```python
from build123d import *

# Parameters (mm, degrees)
EXTRUDE_1_DEPTH   = 5
EXTRUDE_1_2_DEPTH = 5
EXTRUDE_1_3_DEPTH = 3
SKETCH_3_W        = 8
SKETCH_3_H        = 4.5
EXTRUDE_2_DEPTH   = 1
FILLET_1_R        = 2
FILLET_2_R        = 0.4
FILLET_3_R        = 0.4


with BuildPart() as part:
    # Эскиз1 → Extrude 1 (new body)
    with BuildSketch(Plane(origin=(0, 0, 0), x_dir=(1, 0, 0), z_dir=(0, 1, 0))):
        Polygon((3.047071049, 14.786951222), (5.547071049, 14.786951222), (5.547071049, 20.386951222), (-4.052928951, 20.386951222), (-4.052928951, 14.786951222), (-1.552928951, 14.786951222), (-1.552928951, 14.286951222), (3.047071049, 14.286951222), align=None)
        Polygon((2.247071049, 15.586951222), (4.747071049, 15.586951222), (4.747071049, 19.586951222), (-3.252928951, 19.586951222), (-3.252928951, 15.586951222), (-0.752928951, 15.586951222), (-0.752928951, 15.086951222), (2.247071049, 15.086951222), align=None, mode=Mode.SUBTRACT)
    extrude(amount=EXTRUDE_1_DEPTH)



with BuildPart() as body_2:
    # Эскиз1 → Extrude 1 2 (new body)
    with BuildSketch(Plane(origin=(0, 0, 0), x_dir=(1, 0, 0), z_dir=(0, 1, 0))):
        Polygon((-4.052928951, -12.613048778), (-4.052928951, -18.213048778), (5.547071049, -18.213048778), (5.547071049, -12.613048778), (3.047071049, -12.613048778), (3.047071049, -12.113048778), (-1.552928951, -12.113048778), (-1.552928951, -12.613048778), align=None)
        Polygon((-3.252928951, -13.413048778), (-3.252928951, -17.413048778), (4.747071049, -17.413048778), (4.747071049, -13.413048778), (2.247071049, -13.413048778), (2.247071049, -12.913048778), (-0.752928951, -12.913048778), (-0.752928951, -13.413048778), align=None, mode=Mode.SUBTRACT)
    extrude(amount=EXTRUDE_1_2_DEPTH)


with BuildPart() as part_1:
    add(part.part)

    add(body_2.part)  # Extrude 1 3 merges body 2
    # Эскиз2 → Extrude 1 3 (add)
    with BuildSketch(Plane(origin=(0, 5, 0), x_dir=(1, 0, 0), z_dir=(0, 1, 0))):
        Polygon((-4.052928951, 20.386951222), (-13.052928951, 20.386951222), (-13.052928951, -18.213048778), (-4.052928951, -18.213048778), (-4.052928951, -12.613048778), (-8.052928951, -12.613048778), (-8.052928951, 14.786951222), (-4.052928951, 14.786951222), align=None)
    extrude(amount=-EXTRUDE_1_3_DEPTH)

    # Эскиз3 → Бобышка-Вытянуть2 (add)
    with BuildSketch(Plane(origin=(0, 5, 0), x_dir=(1, 0, 0), z_dir=(0, 1, 0))):
        with Locations((0.747071049, 17.336951222)):
            Rectangle(SKETCH_3_W, SKETCH_3_H)
        with Locations((0.747071049, -15.163048778)):
            Rectangle(SKETCH_3_W, SKETCH_3_H)
    extrude(amount=-EXTRUDE_2_DEPTH)

    # Скругление1
    fillet_1_edges = [part_1.edges().sort_by_distance(p)[0] for p in [
        (-4.052928951, 2, -17.586951222),
        (-4.052928951, 2, 15.413048778),
        (-8.052928951, 3.5, 12.613048778),
        (-8.052928951, 3.5, -14.786951222),
        (-13.052928951, 3.5, -20.386951222),
        (-13.052928951, 3.5, 18.213048778),
    ]]
    fillet(fillet_1_edges, radius=FILLET_1_R - 0.0001)  # a hair under: the kernel refuses the full size

    # Скругление2
    fillet_2_edges = [part_1.edges().sort_by_distance(p)[0] for p in [
        (5.547071049, 2.5, -14.786951222),
        (5.547071049, 2.5, -20.386951222),
        (5.547071049, 2.5, 18.213048778),
        (5.547071049, 2.5, 12.613048778),
    ]]
    fillet(fillet_2_edges, radius=FILLET_2_R)

    # Скругление3
    fillet_3_edges = [part_1.edges().sort_by_distance(p)[0] for p in [
        (-0.752928951, 2, -15.586951222),
        (3.047071049, 2.5, -14.786951222),
        (-1.552928951, 2.5, -14.786951222),
        (-0.752928951, 2, 13.413048778),
        (2.247071049, 2, 13.413048778),
        (3.047071049, 2.5, 12.613048778),
        (-1.552928951, 2.5, 12.613048778),
        (2.247071049, 2, -15.586951222),
    ]]
    fillet(fillet_3_edges, radius=FILLET_3_R)


solid = part_1.part
```
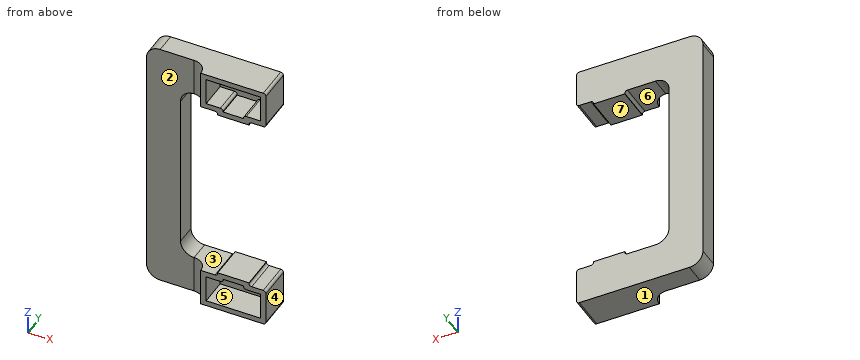
Read the model definition and answer for the solid it produces. Units are mm, in the model's axes. Face numbers are marked on the shaded views. A direction names the side the tool comes from. Give positions to 0.01 mm unless a question says otherwise; leave off trailing zeros. Loops run counter-clockwise (first coordinate to the right, second up) from the corner with the lowest first, then second, coordinate; pieces in that order, holes last.
Item 1: The part is cut by section D-D (y = 1). Give the number of separate pieces and of enclosed holes in the cut face, and give its area (3 significant figures).
Item 2: Each of these flat-tipped pins is pushed along its axis until it touches: pin 1 Ø1 at (y, z) = (4.5, -0.5) entering from +X; pin 2 Ø1.3 at (x, z) = (1.5, 14.5) entering from -Y. Where does it stop, or does it pass through?
Item 3: The part is cut by section A-A (x = 4). Write down the section's boundary in (y, z), and give its area (3 significant figures).
Item 4: For the marked faces 4, 5, 6 and 7, determine the directions among +Z, -Z, +X, -X, +Y, -Y from which every point of the face is accessible in a straight line to the end or side of a thin tool.
Item 5: The mould has two halves that part along Z. Classify the marked faces 1, 2 and 3: released by +Z, released by -Z, zero draft, split by the parting line, or undercut.
Item 6: Find the intervals of material crossed by line 1 along Z through (x, y) = (0, 0.8); line 2 along Z through (x, y) = (3.75, 4.15); line 3 along Z through (x, y) = (3, 4.2), in increasing order.
Item 7: The part is cut by section C-C (x = 0.5). Write down the section's boundary in (y, z).
Taken from the geometry:
1. separate pieces: 2
1. enclosed holes: 2
1. area: 48.0 mm2
2. pin 1: stops at x = -8.05
2. pin 2: stops at y = 4
3. outline: (0, -20.39) - (5, -20.39) - (5, -14.79) - (0, -14.79) - (0, -15.59) - (4, -15.59) - (4, -19.59) - (0, -19.59) - close; (0, 12.61) - (5, 12.61) - (5, 18.21) - (0, 18.21) - (0, 17.41) - (4, 17.41) - (4, 13.41) - (0, 13.41) - close
3. area: 24.0 mm2
4. face 4: +Z, -Z, +X, +Y, -Y
4. face 5: -Y
4. face 6: +Y, -Y
4. face 7: +X, +Y, -Y
5. face 1: released by -Z
5. face 2: zero draft
5. face 3: undercut
6. line 1: z = -20.39 to -19.59, -15.09 to -14.29, 12.11 to 12.91, 17.41 to 18.21
6. line 2: z = -20.39 to -14.79, 12.61 to 18.21
6. line 3: z = -20.39 to -14.29, 12.11 to 18.21
7. outline: (0, -20.39) - (5, -20.39) - (5, -14.29) - (0, -14.29) - (0, -15.09) - (4, -15.09) - (4, -19.59) - (0, -19.59) - close; (0, 12.11) - (5, 12.11) - (5, 18.21) - (0, 18.21) - (0, 17.41) - (4, 17.41) - (4, 12.91) - (0, 12.91) - close
